from build123d import *

# Parameters (mm, degrees)
SKETCH1_R           = 3.175
BOSS_EXTRUDE2_DEPTH = 4.7625
FILLET1_R           = 0.0127


with BuildPart() as part:
    # Sketch1 → Boss-Extrude2 (new body)
    with BuildSketch(Plane.XY):
        with BuildLine():
            Line((131.7244, 0), (87.896637, 4.947593))
            ThreePointArc((87.896637, 4.947593), (88.160392, 4.270718), (88.385012, 3.579871))
            Line((88.385012, 3.579871), (76.2, 6.267993))
            Line((76.2, 6.267993), (-35.963072, 18.929766))
            ThreePointArc((-35.963072, 18.929766), (-26.314005, 14.966389), (-20.198856, 6.515484))
            Line((-20.198856, 6.515484), (-14.231807, 8.687312))
            ThreePointArc((-14.231807, 8.687312), (-14.513112, 9.424368), (-14.81717, 10.152332))
            Line((-14.81717, 10.152332), (-8.496937, 9.438859))
            ThreePointArc((-8.496937, 9.438859), (-12.7, 0), (-8.496937, -9.438859))
            Line((-8.496937, -9.438859), (-14.81717, -10.152332))
            ThreePointArc((-14.81717, -10.152332), (-14.513112, -9.424368), (-14.231807, -8.687312))
            Line((-14.231807, -8.687312), (-20.198856, -6.515484))
            ThreePointArc((-20.198856, -6.515484), (-26.314005, -14.966389), (-35.963072, -18.929766))
            Line((-35.963072, -18.929766), (76.2, -6.267993))
            Line((76.2, -6.267993), (88.385012, -3.579871))
            ThreePointArc((88.385012, -3.579871), (88.160392, -4.270718), (87.896637, -4.947593))
            Line((87.896637, -4.947593), (131.7244, 0))
        make_face()
        Circle(SKETCH1_R, mode=Mode.SUBTRACT)
        with BuildLine():
            Line((75.116267, 0), (10.387338, 7.307066))
            ThreePointArc((10.387338, 7.307066), (12.7, 0), (10.387338, -7.307066))
            Line((10.387338, -7.307066), (75.116267, 0))
        make_face(mode=Mode.SUBTRACT)
    extrude(amount=-BOSS_EXTRUDE2_DEPTH)

    # Fillet1
    fillet1_edges = [part.edges().sort_by_distance(p)[0] for p in [
        (-35.963072, 18.929766, -2.38125),
        (-35.963072, -18.929766, -2.38125),
    ]]
    fillet(fillet1_edges, radius=FILLET1_R)


solid = part.part
Build history of the part. All positions in model axes, mm. A direction names the side the tool comes from. Round coordinates to 2 decimals unless told otherwise and drop trailing zeros. Loops run counter-clockwise (first coordinate to the right, second up) from the corner with the lowest first, then second, coordinate; pieces in that order, holes last. Notation, with made-up numbers: (29.5, 53) -> (43.5, 53) arc R20 ccw to (43.5, 78) -> close; hole circle Ø3 at (77, 47). An arc over 180 degrees is marked (long way). Answer in a Markdown table with one row per item.
Item 1: Drill centre lines: L1, parallel to Y at x = -9, z = -2.8; L2, parallel to Y at x = 0, z = -3.8 (3 decimals); L3, parallel to Y at x = -10, z = -2.95. Where is each one in solid material? Low to high. Write a range as [from, to].
Answers below:
| item | result |
|---|---|
| L1 | y = [-15.89, -9.5], [-8.96, 8.96], [9.5, 15.89] |
| L2 | y = [-14.87, -3.175], [3.175, 14.87] |
| L3 | y = [-16, -9.61], [-7.83, 7.83], [9.61, 16] |
Item 2: Pin check, flat tip, straight feed: pin 1 (1 mm diameter, centred on x = 56, z = -2, fed in from -Y). Stop position of the tip, or through.
Answers below:
| item | result |
|---|---|
| pin 1 | stops at y = -8.6 |
Item 3: Which spindle directions (+Z, -Z, +X, -X, +Y, -Y) get a long thin tool onto all of the face, cutting with end or side? Do faces 1 (the cylindrical face through (-26.04, 14.747, -2.348)), 2 (the flat face through (42.299, -3.705, -2.348)), 3 (the flat face through (109.5, -2.51, -2.35)). Say none if no direction does.
Answers below:
| item | result |
|---|---|
| face 1 | +Z, -Z, -X |
| face 2 | +Z, -Z |
| face 3 | +Z, -Z, +X, -Y |
Item 4: Saw through at C-C (y = -1.5). Write the cut outline in (x, z).
Answers below:
| item | result |
|---|---|
| outline | (-12.61, -4.76) -> (-2.8, -4.76) -> (-2.8, 0) -> (-12.61, 0) -> close; (2.8, -4.76) -> (12.61, -4.76) -> (12.61, 0) -> (2.8, 0) -> close; (61.83, -4.76) -> (118.44, -4.76) -> (118.44, 0) -> (61.83, 0) -> close |
Item 5: Saw through at D-D (x = 26.5). Write the cut outline in (y, z), and give its area (3 significant figures).
Answers below:
| item | result |
|---|---|
| outline | (-11.88, -4.76) -> (-5.49, -4.76) -> (-5.49, 0) -> (-11.88, 0) -> close; (5.49, -4.76) -> (11.88, -4.76) -> (11.88, 0) -> (5.49, 0) -> close |
| area | 60.9 mm² |
Item 6: Saw through at B-B (x = 0). Write the cut outline in (y, z) (1 decimal).
Answers below:
| item | result |
|---|---|
| outline | (-14.9, -4.8) -> (-3.2, -4.8) -> (-3.2, 0) -> (-14.9, 0) -> close; (3.2, -4.8) -> (14.9, -4.8) -> (14.9, 0) -> (3.2, 0) -> close |
Item 7: Mould opens along Y. For faces 4 (the cylindrical face through (-25.823, -14.567, -2.348)), 5 (the flat face through (36, -5, -4.762)), 6 (the flat face through (110.12, 2.44, -2.35)) say: +Y half, -Y half, draft (parallel to the pull), parting line (faces both ways), or undercut.
Answers below:
| item | result |
|---|---|
| face 4 | undercut |
| face 5 | draft |
| face 6 | +Y half |
Item 8: Saw through at A-A (z = -0.85). Write the cut outline in (x, y) (3 decimals).
Answers below:
| item | result |
|---|---|
| outline | (-34.989, -18.794) arc R0.013 ccw to (-34.986, -18.819) -> (76.2, -6.268) -> (88.385, -3.58) arc R12.7 cw to (87.897, -4.948) -> (131.724, 0) -> (87.897, 4.948) arc R12.7 cw to (88.385, 3.58) -> (76.2, 6.268) -> (-34.986, 18.819) arc R0.013 ccw to (-34.989, 18.794) arc R19.05 cw to (-20.199, 6.515) -> (-14.232, 8.687) arc R25.401 ccw to (-14.817, 10.152) -> (-8.497, 9.439) arc R12.7 ccw to (-8.497, -9.439) -> (-14.817, -10.152) arc R25.401 ccw to (-14.232, -8.687) -> (-20.199, -6.515) arc R19.05 cw to start; hole circle Ø6.35 at (0, 0); hole (10.387, -7.307) -> (75.116, 0) -> (10.387, 7.307) arc R12.7 cw to start |
